Could you check a few things on this model? Use its own coordinates, in mm. Face numbers are marked on the shaded views. A direction names the side the tool comes from. Give positions to 0.01 mm unless a question says otherwise; leave off trailing zeros. Loops run counter-clockwise (first coordinate to the right, second up) from the corner with the lowest first, then second, coordinate; pieces in that order, holes last.
1. Imagine slicing it at B-B (y = -5.75). List the corners of the cut face in (x, z) for me, plus the area to 3 significant figures.
2. Imagine slicing it at D-D (z = 14). Count the separate pieces of the cut face and the enclosed holes in it, plus the area to 3 significant figures.
3. Imagine slicing it at A-A (z = 7). List the corners of the cut face in (x, y) for me, plus the area to 3 significant figures.
4. I need wall thicknesses on line 1 along X through (y, z) = (5.8, 4.5); line 2 along X through (y, z) = (3.25, 11.5); line 3 along Y through (x, z) = (17, 11.5). Which ranges of each line are inside material? Lowest first, please.
5. For P1, Ø6, axis at x = 25.5, z = 13, coming from the -Y side; P2, Ø3, axis at x = -7.5, z = 13, coming from the -Y side; P3, Ø2.5, axis at y = -1.5, z = 10.5, coming from the -X side, each with a flat end and sliding along its axis, tell me the tip position at first contact or that it passes through.
6. Thinking about a two-plate mould opening in X: for the marked faces 5, 6, 7 and 8, which applies, +X half, -X half, draft (parallel to the pull), parting line (faces both ways), or undercut?
7. For the marked faces 1, 2, 3 and 4, which set-ups out of +Z, -Z, +X, -X, +Y, -Y let a thin tool reach every point of the face, with its end or its side?
```python
from build123d import *

# Parameters (mm, degrees)
F1_DEPTH    = 15.7
F2_W        = 10.0960650777
F2_H        = 2.35
F3_DEPTH    = 8
F4_R        = 5
F5_T1_DEPTH = 26.8923143391
F5_T3_DEPTH = 21.3473434867
F5_T5_DEPTH = 35.7
F6_W        = 15
F6_H        = 6.25
F7_DEPTH    = 2
F8_SIZE     = 1.99999


# Not quite as in the source:
# - a fillet or chamfer that OpenCascade refuses, or shapes differently, is made with other operations: its cross-section is extruded or revolved along the edge and cut away or added
# - a fillet or chamfer is up to 0.001 mm smaller than in the source, because OpenCascade refuses the exact size


with BuildPart() as f1:
    # F0 (on Top) → F1 (new body)
    with BuildSketch(Plane.XY):
        Polygon((30, 9), (0, 9), (0, -1.8), (15, -1.8), (15, -9), (19.5954625243, -9), (30, -2.6151265483), align=None)
        with BuildLine():
            ThreePointArc((21.17, -5.2), (17.9264971157, -6.5435028843), (19.27, -3.3))
            ThreePointArc((19.27, -3.3), (20.6135028843, -3.8564971157), (21.17, -5.2))
        make_face(mode=Mode.SUBTRACT)
        with BuildLine():
            ThreePointArc((19.27, 3.9), (17.9264971157, 7.1435028843), (21.17, 5.8))
            ThreePointArc((21.17, 5.8), (20.6135028843, 4.4564971157), (19.27, 3.9))
        make_face(mode=Mode.SUBTRACT)
        with BuildLine():
            ThreePointArc((24.47, 5.8), (26.37, 7.7), (28.27, 5.8))
            ThreePointArc((28.27, 5.8), (26.37, 3.9), (24.47, 5.8))
        make_face(mode=Mode.SUBTRACT)
    extrude(amount=F1_DEPTH)

    # F2 (on face) → F3 (cut)
    with BuildSketch(Plane.XY.offset(15.7)):
        with BuildLine():
            ThreePointArc((11.6039349223, -0.1749693412), (8.8681704068, 4.0561246908), (13.8492571677, 4.8146356484))
            Line((13.8492571677, 4.8146356484), (16.291649806, 2.0583304766))
            ThreePointArc((16.291649806, 2.0583304766), (16.3383380366, 2.4404176698), (16.3539349223, 2.8250306588))
            ThreePointArc((16.3539349223, 2.8250306588), (16.0600367861, 4.4699185515), (15.2147112678, 5.9112571869))
            ThreePointArc((15.2147112678, 5.9112571869), (7.5463441808, 5.2945361506), (10.5215341623, -1.8))
            Line((10.5215341623, -1.8), (12.6863356823, -1.8))
            ThreePointArc((12.6863356823, -1.8), (14.1212348386, -1.2030831841), (15.286664888, -0.1749693412))
            Line((15.286664888, -0.1749693412), (11.6039349223, -0.1749693412))
        make_face()
        with BuildLine():
            ThreePointArc((16.3539349223, 2.8250306588), (16.3383380366, 2.4404176698), (16.291649806, 2.0583304766))
            Line((16.291649806, 2.0583304766), (17.1652654837, 1.0724319062))
            ThreePointArc((17.1652654837, 1.0724319062), (17.3051830671, 0.8410213344), (17.3539349223, 0.5750306588))
            ThreePointArc((17.3539349223, 0.5750306588), (17.1342650082, 0.0447005729), (16.6039349223, -0.1749693412))
            Line((16.6039349223, -0.1749693412), (15.286664888, -0.1749693412))
            ThreePointArc((15.286664888, -0.1749693412), (14.1212348386, -1.2030831841), (12.6863356823, -1.8))
            Line((12.6863356823, -1.8), (15, -1.8))
            Line((15, -1.8), (15, -1.9249693412))
            Line((15, -1.9249693412), (19.9039349223, -1.9249693412))
            Line((19.9039349223, -1.9249693412), (19.9039349223, 0.4250306588))
            Line((19.9039349223, 0.4250306588), (15.2147112678, 5.9112571869))
            ThreePointArc((15.2147112678, 5.9112571869), (16.0600367861, 4.4699185515), (16.3539349223, 2.8250306588))
        make_face()
        with Locations((24.9519674612, -0.7499693412)):
            Rectangle(F2_W, F2_H)
    extrude(amount=-F3_DEPTH, mode=Mode.SUBTRACT)

    # F4
    f4_edges = [f1.edges().sort_by_distance(p)[0] for p in [
        (19.903935, 0.425031, 11.7),
    ]]
    fillet(f4_edges, radius=F4_R)

    # F5: fillet of radius 4 on 4 edges, made by hand

    # F5_s2 → F5_t1 (cut)
    with BuildSketch(Plane.XY.offset(-5.5961571696)):
        with BuildLine():
            ThreePointArc((30, -0.3766636805), (29.4905957559, -2.3300559271), (28.0921293656, -3.7859150232))
            Line((28.0921293656, -3.7859150232), (30, -2.6151265483))
            Line((30, -2.6151265483), (30, -0.3766636805))
        make_face()
    extrude(amount=F5_T1_DEPTH, mode=Mode.SUBTRACT)

    # F5_s4 → F5_t3 (cut)
    with BuildSketch(Plane.XY.offset(-2.8236717433)):
        with BuildLine():
            ThreePointArc((20.5581231925, -8.4092513427), (19.5529608525, -8.8494808332), (18.465993827, -9))
            Line((18.465993827, -9), (19.5954625243, -9))
            Line((19.5954625243, -9), (20.5581231925, -8.4092513427))
        make_face()
    extrude(amount=F5_T3_DEPTH, mode=Mode.SUBTRACT)

    # F5_s6 → F5_t5 (cut)
    with BuildSketch(Plane.XY.offset(-10)):
        with BuildLine():
            ThreePointArc((15, -5), (16.1715728753, -7.8284271247), (19, -9))
            Line((19, -9), (15, -9))
            Line((15, -9), (15, -5))
        make_face()
        with BuildLine():
            ThreePointArc((30, 5), (28.8284271247, 7.8284271247), (26, 9))
            Line((26, 9), (30, 9))
            Line((30, 9), (30, 5))
        make_face()
    extrude(amount=F5_T5_DEPTH, mode=Mode.SUBTRACT)

    # F6 (on face) → F7 (cut)
    with BuildSketch(Plane.XZ.offset(1.8)):
        with Locations((7.5, 3.125)):
            Rectangle(F6_W, F6_H)
    extrude(amount=-F7_DEPTH, mode=Mode.SUBTRACT)

    # F8 (size 2 in the source; OpenCascade refuses exactly that, so slightly less here)
    f8_edges = [f1.edges().sort_by_distance(p)[0] for p in [
        (7.5, 0.2, 6.25),
    ]]
    chamfer(f8_edges, length=F8_SIZE)

    # F9: F1 across plane


with BuildPart() as f1_1:
    add(f1.part)
    add(f1.part.mirror(Plane.YZ))


solid = f1_1.part
```
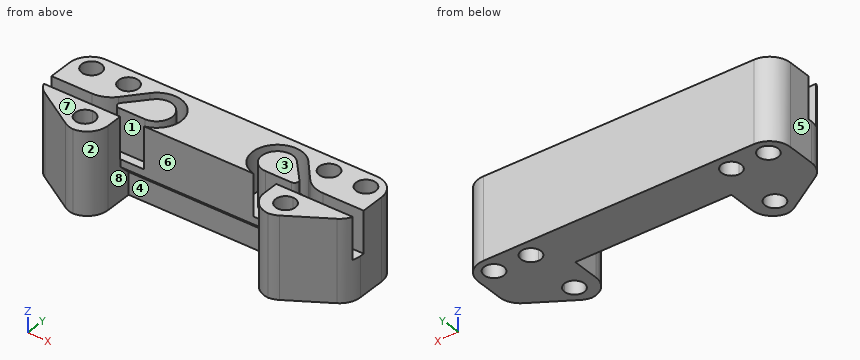
Derived:
1. outline: (-24.89, 0) - (-21.09, 0) - (-21.09, 15.7) - (-24.89, 15.7) - close; (-17.45, 0) - (-15.07, 0) - (-15.07, 15.7) - (-17.45, 15.7) - close; (15.07, 0) - (17.45, 0) - (17.45, 15.7) - (15.07, 15.7) - close; (21.09, 0) - (24.89, 0) - (24.89, 15.7) - (21.09, 15.7) - close
1. area: 194 mm2
2. separate pieces: 5
2. enclosed holes: 6
2. area: 558 mm2
3. outline: (-30, -0.38) arc R4 ccw to (-28.09, -3.79) - (-20.56, -8.41) arc R4 ccw to (-18.73, -8.99) arc R4 ccw to (-15, -5) - (-15, -1.8) - (15, -1.8) - (15, -5) arc R4 ccw to (18.73, -8.99) arc R4 ccw to (20.56, -8.41) - (28.09, -3.79) arc R4 ccw to (30, -0.38) - (30, 5) arc R4 ccw to (26, 9) - (-26, 9) arc R4 ccw to (-30, 5) - close; hole circle Ø3.8 at (-26.37, 5.8); hole circle Ø3.8 at (-19.27, -5.2); hole circle Ø3.8 at (-19.27, 5.8); hole circle Ø3.8 at (19.27, -5.2); hole circle Ø3.8 at (19.27, 5.8); hole circle Ø3.8 at (26.37, 5.8)
3. area: 714 mm2
4. line 1: x = -29.92 to -28.27, -24.47 to -21.17, -17.37 to 17.37, 21.17 to 24.47, 28.27 to 29.92
4. line 2: x = -30 to -17.49, -15.24 to -8.63, -6.87 to 6.87, 8.63 to 15.24, 17.49 to 30
4. line 3: y = -8.46 to -1.92, -0.06 to 1.26, 3.82 to 9
5. P1: stops at y = -7.22
5. P2: stops at y = -1.8
5. P3: stops at x = -29.69
6. face 5: -X half
6. face 6: undercut
6. face 7: draft
6. face 8: undercut
7. face 1: +Z, -X
7. face 2: +Z, -Z, -Y
7. face 3: +Z, +X, -X, +Y, -Y
7. face 4: -Z, -Y
